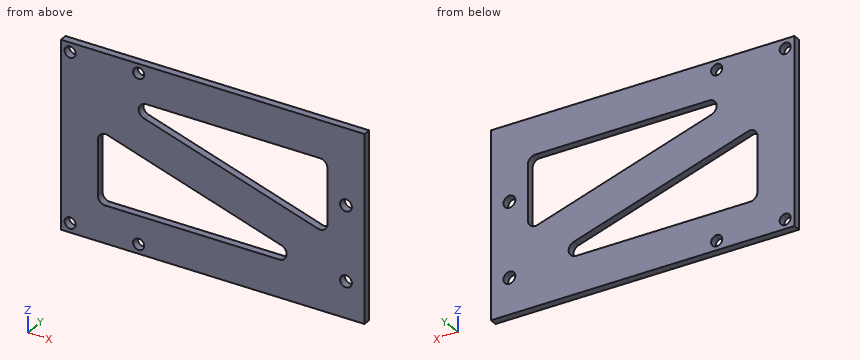
from build123d import *

# Parameters (mm, degrees)
SKETCH_1_W          = 82
SKETCH_1_H          = 50
SKETCH_1_R          = 1.5
EXTRUDE_1_DEPTH     = 2
SKETCH_2_R          = 1.6
CUT_EXTRUDE_1_DEPTH = 2
CUT_EXTRUDE_2_DEPTH = 2
FILLET_1_R          = 2


with BuildPart() as part:
    # 草图1 → 凸台-拉伸1 (new body)
    with BuildSketch(Plane(origin=(0, 0, 0), x_dir=(1, 0, 0), z_dir=(0, 1, 0))):
        with Locations((41, 25)):
            Rectangle(SKETCH_1_W, SKETCH_1_H)
        with Locations(Location((2.5, 47.5, 0), (0, 0, 270))):
            Circle(SKETCH_1_R, mode=Mode.SUBTRACT)
        with Locations(Location((2.5, 2.5, 0), (0, 0, 270))):
            Circle(SKETCH_1_R, mode=Mode.SUBTRACT)
        with Locations(Location((21, 47.5, 0), (0, 0, 270))):
            Circle(SKETCH_1_R, mode=Mode.SUBTRACT)
        with Locations(Location((21, 2.5, 0), (0, 0, 270))):
            Circle(SKETCH_1_R, mode=Mode.SUBTRACT)
    extrude(amount=EXTRUDE_1_DEPTH)

    # 草图2 → 切除-拉伸1 (cut)
    with BuildSketch(Plane(origin=(0, 2, 0), x_dir=(1, 0, 0), z_dir=(0, 1, 0))):
        with Locations(Location((77, 20.3, 0), (0, 0, 270))):
            Circle(SKETCH_2_R)
        with Locations(Location((77, 40.3, 0), (0, 0, 270))):
            Circle(SKETCH_2_R)
    extrude(amount=-CUT_EXTRUDE_1_DEPTH, mode=Mode.SUBTRACT)

    # 草图4 → 切除-拉伸2 (cut)
    with BuildSketch(Plane(origin=(0, 2, 0), x_dir=(1, 0, 0), z_dir=(0, 1, 0))):
        Polygon((10, 10), (72, 10), (72, 29.516271877), align=None)
        Polygon((10, 20.483728123), (10, 40), (72, 40), align=None)
    extrude(amount=-CUT_EXTRUDE_2_DEPTH, mode=Mode.SUBTRACT)

    # 圆角1
    fillet_1_edges = [part.edges().sort_by_distance(p)[0] for p in [
        (72, 1, -40),
        (10, 1, -20.483728123),
        (10, 1, -40),
        (10, 1, -10),
        (72, 1, -29.516271877),
        (72, 1, -10),
    ]]
    fillet(fillet_1_edges, radius=FILLET_1_R)


solid = part.part
Read the model definition and answer for the solid it produces. Units are mm, in the model's axes. Give positions to 0.01 mm unless a question says otherwise; leave off trailing zeros. Write each loop counter-clockwise with the first axis right and the second up, starting at its lowest first coordinate (ties: lowest second). Pieces come first, ordered by that corner, then holes. Notation, with made-up numbers: (-18, 13) - (-6, 13) arc R8 ccw to (-6, 28) - close; hole circle Ø4 at (-15.5, 26). An arc over 180 degrees is marked (long way). Answer in a Markdown table with one row per item. Add a question column.
Item 1: Flat-ended cylindrical pins translate along their axes: P1, Ø1, axis at y = 0.5, z = -19, coming from the -X side; P2, Ø1.8, axis at x = 21, z = -2.5, coming from the +Y side. Find the tip coordinate at first contact, or state that the pin passes through.
Item 2: Section D-D, the plane x = 62.5 is taken. Write down the section's boundary in (y, z).
Item 3: Find the intervals of material crossed by L1, parallel to X at y = 1.1, z = -47.5; L2, parallel to Z at x = 77, y = 1.15; L3, parallel to X at y = 1.4, z = -40.3, in increasing order.
Item 4: Section A-A, the plane y = 0.8 is taken. Count the separate pieces of the cut face and the enclosed holes in it, and give its area (3 significant figures).
Item 5: Section C-C, the plane z = -2.5 is taken. Write down the section's boundary in (x, y), and give its area (3 significant figures).
Item 6: Section B-B, the plane x = 2.5 is taken. Write down the section's boundary in (y, z), and give its area (3 significant figures).
Recorded:
| question | item | result |
|---|---|---|
| 1 | P1 | stops at x = 0 |
| 1 | P2 | passes through |
| 2 | outline | (0, -50) - (2, -50) - (2, -26.53) - (0, -26.53) - close; (0, -10) - (2, -10) - (2, 0) - (0, 0) - close |
| 3 | L1 | x = 0 to 1, 4 to 19.5, 22.5 to 82 |
| 3 | L2 | z = -50 to -41.9, -38.7 to -21.9, -18.7 to 0 |
| 3 | L3 | x = 0 to 75.4, 78.6 to 82 |
| 4 | separate pieces | 1 |
| 4 | enclosed holes | 8 |
| 4 | area | 2,890 mm2 |
| 5 | outline | (0, 0) - (1, 0) - (1, 2) - (0, 2) - close; (4, 0) - (19.5, 0) - (19.5, 2) - (4, 2) - close; (22.5, 0) - (82, 0) - (82, 2) - (22.5, 2) - close |
| 5 | area | 152 mm2 |
| 6 | outline | (0, -50) - (2, -50) - (2, -49) - (0, -49) - close; (0, -46) - (2, -46) - (2, -4) - (0, -4) - close; (0, -1) - (2, -1) - (2, 0) - (0, 0) - close |
| 6 | area | 88.0 mm2 |
